Geometry check sheet. Reference: the model listing, model coordinates, mm. Face numbers are marked on the shaded views. A direction names the side the tool comes from. Round coordinates to 2 decimals unless told otherwise and drop trailing zeros. Order: outer loops, then holes, each group sorted by start corner. A loop starts at its lowest first (then second) coordinate and runs counter-clockwise, first axis right, second up. Notation, with made-up numbers: (69, 56.5) -> (110, 56.5) arc R16 cw to (110, 69.5) -> close; hole circle Ø2 at (61.25, -29.75). An arc over 180 degrees is marked (long way). Use a Markdown table: item, result. Add a question column.
Item 1: Sectioned sample at A-A, the plane y = 1.75. Record the cut outline in (x, z), and give its area (3 significant figures).
Item 2: Sectioned sample at D-D, the plane x = 18. Record the cut outline in (y, z).
Item 3: Sectioned sample at B-B, the plane z = -6.5. Record the cut outline in (x, y), and give its area (3 significant figures).
Item 4: Material ranges on probe 1 along Z at (x, y) = (5, 1.4); probe 2 along Z at (x, y) = (5, 3.85); probe 3 along Z at (x, y) = (19.5, 12.25), recorded low to high. Write a range as [from, to].
Item 5: Gauge pin test, flat ends, axial feed: pin 1 Ø4 at (x, y) = (16.5, 11) entering from -Z; pin 2 Ø6.5 at (x, y) = (6.5, 10) entering from -Z; pin 3 Ø5.5 at (x, y) = (-5.5, 10) entering from +Z; pin 4 Ø1 at (x, y) = (12, 7) entering from +Z. Record the tip position at first contact, or that the pin passes through.
Item 6: Set-up check for the marked faces 1, 2, 3 and 4: record each of +Z, -Z, +X, -X, +Y, -Y from which the full face is reachable in a straight line by a thin tool's end or side.
Item 7: Sectioned sample at C-C, the plane y = 10.75. Record the cut outline in (x, z), and give its area (3 significant figures).
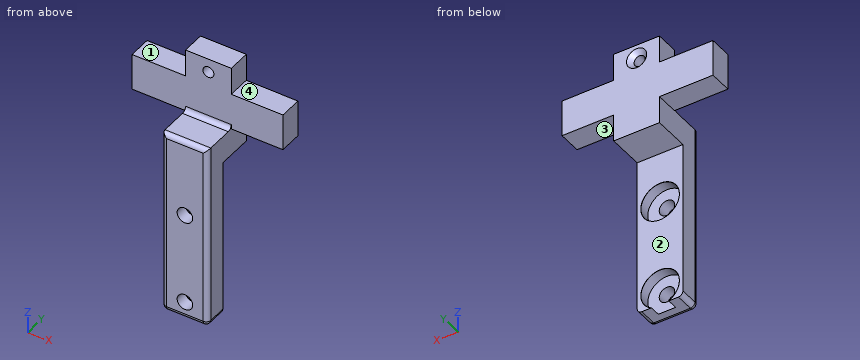
from build123d import *

# Parameters (mm, degrees)
SKETCH1_W                                       = 10
SKETCH1_H                                       = 40.8
BOSS_EXTRUDE1_DEPTH                             = 5
SKETCH7_W                                       = 10
SKETCH7_H                                       = 6
BOSS_EXTRUDE2_DEPTH                             = 7.83
SKETCH8_W                                       = 33
SKETCH8_H                                       = 5
BOSS_EXTRUDE3_DEPTH                             = 8
SKETCH9_W                                       = 10
SKETCH9_H                                       = 5
BOSS_EXTRUDE4_DEPTH                             = 6
CSK_FOR_M2_FLAT_HEAD_MACHINE_SCREW1_D           = 2.4
CSK_FOR_M2_FLAT_HEAD_MACHINE_SCREW1_CSINK_D     = 4.4
CSK_FOR_M2_FLAT_HEAD_MACHINE_SCREW1_CSINK_ANGLE = 90
CBORE_FOR_M3_HEX_HEAD_MACHINE_SCREW1_AT_COUNT   = 2
CBORE_FOR_M3_HEX_HEAD_MACHINE_SCREW1_AT_PITCH   = 20
FILLET1_R                                       = 1


with BuildPart() as part:
    # Sketch1 → Boss-Extrude1 (new body)
    with BuildSketch(Plane(origin=(0, 0, 0), x_dir=(1, 0, 0), z_dir=(0, 1, 0))):
        with Locations((5, 24.563754531)):
            Rectangle(SKETCH1_W, SKETCH1_H)
    extrude(amount=BOSS_EXTRUDE1_DEPTH)

    # Sketch7 → Boss-Extrude2 (add)
    with BuildSketch(Plane(origin=(0, 5, 0), x_dir=(1, 0, 0), z_dir=(0, 1, 0))):
        with Locations((5, 7.163754531)):
            Rectangle(SKETCH7_W, SKETCH7_H)
    extrude(amount=BOSS_EXTRUDE2_DEPTH)

    # Sketch8 → Boss-Extrude3 (add)
    with BuildSketch(Plane.XY.offset(-4.163754531)):
        with Locations((4.8, 10.33)):
            Rectangle(SKETCH8_W, SKETCH8_H)
    extrude(amount=BOSS_EXTRUDE3_DEPTH)

    # Sketch9 → Boss-Extrude4 (add)
    with BuildSketch(Plane.XY.offset(3.836245469)):
        with Locations((5, 10.33)):
            Rectangle(SKETCH9_W, SKETCH9_H)
    extrude(amount=BOSS_EXTRUDE4_DEPTH)

    # CSK for M2 Flat Head Machine Screw1 (through all)
    with Locations(Plane(origin=(0, 12.83, 0), x_dir=(1, 0, 0), z_dir=(0, 1, 0))):
        with Locations((5, -6.836245469)):
            CounterSinkHole(CSK_FOR_M2_FLAT_HEAD_MACHINE_SCREW1_D / 2, CSK_FOR_M2_FLAT_HEAD_MACHINE_SCREW1_CSINK_D / 2, counter_sink_angle=CSK_FOR_M2_FLAT_HEAD_MACHINE_SCREW1_CSINK_ANGLE)

    # Sketch13 → CBORE for M3 Hex Head Machine Screw1 (revolve, cut)
    with BuildSketch(Plane(origin=(5, 5, -21.213754531), x_dir=(0, 0, 1), z_dir=(1, 0, 0))):
        Polygon((0, 0), (0, 5), (1.7, 5), (1.7, 2.3), (4.2, 2.3), (4.2, 0.025), (4.225, 0), align=None)
    cbore_for_m3_hex_head_machine_screw1 = revolve(axis=Axis((5, 11.35, -21.213754531), (0, -1, 0)), mode=Mode.SUBTRACT)

    # CBORE for M3 Hex Head Machine Screw1 at: CBORE for M3 Hex Head Machine Screw1 ×2
    with Locations(*[(0, 0, -i * CBORE_FOR_M3_HEX_HEAD_MACHINE_SCREW1_AT_PITCH) for i in range(1, CBORE_FOR_M3_HEX_HEAD_MACHINE_SCREW1_AT_COUNT)]):
        add(cbore_for_m3_hex_head_machine_screw1, mode=Mode.SUBTRACT)

    # Fillet1
    fillet1_edges = [part.edges().sort_by_distance(p)[0] for p in [
        (5, 7.83, -4.163754531),
        (5, 0, -44.963754531),
        (10, 0, -24.563754531),
        (5, 0, -4.163754531),
        (0, 0, -24.563754531),
        (0, 2.5, -44.963754531),
        (10, 2.5, -44.963754531),
    ]]
    fillet(fillet1_edges, radius=FILLET1_R)


solid = part.part
Found:
| question | item | result |
|---|---|---|
| 1 | outline | (0, -43.96) arc R1 ccw to (1, -44.96) -> (9, -44.96) arc R1 ccw to (10, -43.96) -> (10, -4.16) -> (0, -4.16) -> close; hole circle Ø3.4 at (5, -41.21); hole circle Ø3.4 at (5, -21.21) |
| 1 | area | 389 mm2 |
| 2 | outline | (7.83, -4.16) -> (12.83, -4.16) -> (12.83, 3.84) -> (7.83, 3.84) -> close |
| 3 | outline | (0, 1) arc R1 ccw to (1, 0) -> (9, 0) arc R1 ccw to (10, 1) -> (10, 12.83) -> (0, 12.83) -> close |
| 3 | area | 128 mm2 |
| 4 | probe 1 | z = [-44.96, -42.91], [-39.51, -22.91], [-19.51, -4.16] |
| 4 | probe 2 | z = [-37.01, -25.41], [-17.01, -4.16] |
| 4 | probe 3 | z = [-4.16, 3.84] |
| 5 | pin 1 | stops at z = -4.16 |
| 5 | pin 2 | stops at z = -10.16 |
| 5 | pin 3 | stops at z = 3.84 |
| 5 | pin 4 | passes through |
| 6 | face 1 | +Z, -X, +Y, -Y |
| 6 | face 2 | -Z, +X, -X, +Y |
| 6 | face 3 | -Z, +X, +Y, -Y |
| 6 | face 4 | +Z, +X, +Y, -Y |
| 7 | outline | (-11.7, -4.16) -> (0, -4.16) -> (0, -10.16) -> (10, -10.16) -> (10, -4.16) -> (21.3, -4.16) -> (21.3, 3.84) -> (10, 3.84) -> (10, 9.84) -> (0, 9.84) -> (0, 3.84) -> (-11.7, 3.84) -> close; hole circle Ø2.4 at (5, 6.84) |
| 7 | area | 379 mm2 |
